```python
from build123d import *

# Parameters (mm, degrees)
BOSS_EXTRUDE3_DEPTH = 1.5875
SKETCH4_R           = 7.14375
BOSS_EXTRUDE4_DEPTH = 19.05
BOSS_EXTRUDE4_TAPER = 1.3
SKETCH5_R           = 1.5875
CUT_EXTRUDE1_DEPTH  = 43.693126115


with BuildPart() as part:
    # Sketch3 → Boss-Extrude3 (new body)
    with BuildSketch(Plane(origin=(0, 0, 0), x_dir=(1, 0, 0), z_dir=(0, 1, 0))):
        Polygon((8.248891971, 0), (4.124445986, 7.14375), (-4.124445986, 7.14375), (-8.248891971, 0), (-4.124445986, -7.14375), (4.124445986, -7.14375), align=None)
    boss_extrude3 = extrude(amount=BOSS_EXTRUDE3_DEPTH)

    # Sketch4 → Boss-Extrude4 (add)
    with BuildSketch(Plane(origin=(0, 1.5875, 0), x_dir=(1, 0, 0), z_dir=(0, 1, 0))):
        Circle(SKETCH4_R)
    boss_extrude4 = extrude(amount=BOSS_EXTRUDE4_DEPTH, taper=BOSS_EXTRUDE4_TAPER)

    # Mirror1: Boss-Extrude3, Boss-Extrude4 across plane
    add(boss_extrude3.mirror(Plane.ZX))
    add(boss_extrude4.mirror(Plane.ZX))

    # Sketch5 → Cut-Extrude1 (cut, through all)
    with BuildSketch(Plane(origin=(0, 20.6375, 0), x_dir=(1, 0, 0), z_dir=(0, 1, 0))):
        with Locations(Location((0, 0, 0), (0, 0, 270))):
            Circle(SKETCH5_R)
    extrude(amount=-CUT_EXTRUDE1_DEPTH, mode=Mode.SUBTRACT)


solid = part.part
```
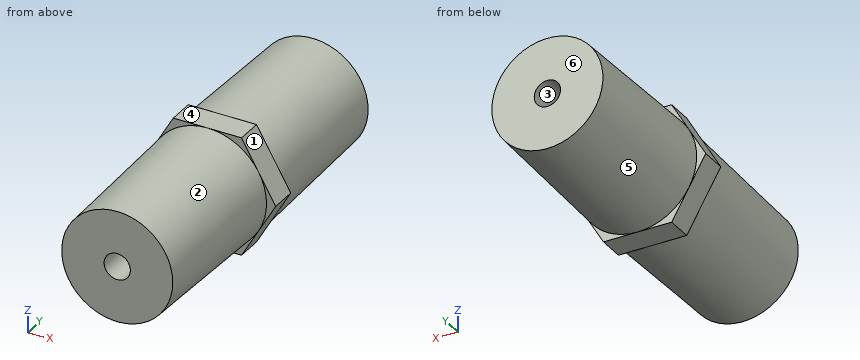
CAD build for the part. Positions are in the model's coordinates, mm. Face numbers are marked on the shaded views. A direction names the side the tool comes from. Coordinates: 2 decimals unless noted, no trailing zeros. Write each loop counter-clockwise with the first axis right and the second up, starting at its lowest first coordinate (ties: lowest second). Pieces come first, ordered by that corner, then holes. Notation, with made-up numbers: (-14, 28.25) -> (13, 28.25) arc R24 cw to (13, 46.25) -> close; hole circle Ø10 at (78, -12). An arc over 180 degrees is marked (long way). Use CSV: the item, a comma, the result in double quotes. Start each with the question number.
Item 1: Tool access for the marked faces 1 and 2: list every direction of +Z, -Z, +X, -X, +Y, -Y with a clear straight run to the whole face (end or side of a thin tool).
Item 2: Wall check: probe 1 along X at (y, z) = (1, 0); probe 2 along X at (y, z) = (-12, -0.75); probe 3 along Y at (x, z) = (-5.25, 5). Give the ranges that are in metal, low to high.
Item 3: Band-saw the part on B-B, the plane y = -11. Write the cut outline in (x, z) (1 decimal), plus the area to 3 significant figures.
Item 4: Band-saw the part on A-A, the plane y = -0.5. Write the cut outline in (x, z) (1 decimal).
Item 5: Band-saw the part on C-C, the plane y = 18. Write the cut outline in (x, z) (1 decimal).
Item 6: Two-plate mould, pull along Z, no slides. Class the marked faces 3, 4, 5 and 6: +Z half, -Z half, draft (parallel to the pull), parting line (faces both ways), or undercut.
Item 7: Drop flat-ended pins along their axis: P1, Ø2, axis at x = -1.5, y = 8.5, coming from the +Z side; P2, Ø8, axis at x = 2, y = 7, coming from the -Z side; P3, Ø5, axis at x = -5, z = -5, coming from the -Y side; P4, Ø3, axis at y = 12, z = 0, coming from the -X side. Give the stop position or say it passes through.
Response values:
1,face 1,"+Z, +X, +Y, -Y"
1,face 2,"-Y"
2,probe 1,"x = -8.25 to -1.59, 1.59 to 8.25"
2,probe 2,"x = -6.87 to -1.4, 1.4 to 6.87"
2,probe 3,"y = -1.59 to 1.59"
3,outline,"circle Ø13.9 at (0, 0); hole circle Ø3.2 at (0, 0)"
3,area,"143 mm2"
4,outline,"(-8.2, 0) -> (-4.1, -7.1) -> (4.1, -7.1) -> (8.2, 0) -> (4.1, 7.1) -> (-4.1, 7.1) -> close; hole circle Ø3.2 at (0, 0)"
5,outline,"circle Ø13.5 at (0, 0); hole circle Ø3.2 at (0, 0)"
6,face 3,"undercut"
6,face 4,"+Z half"
6,face 5,"parting line"
6,face 6,"draft"
7,P1,"stops at z = 6.97"
7,P2,"stops at z = -7.1"
7,P3,"stops at y = -20.64"
7,P4,"stops at x = -6.94"
